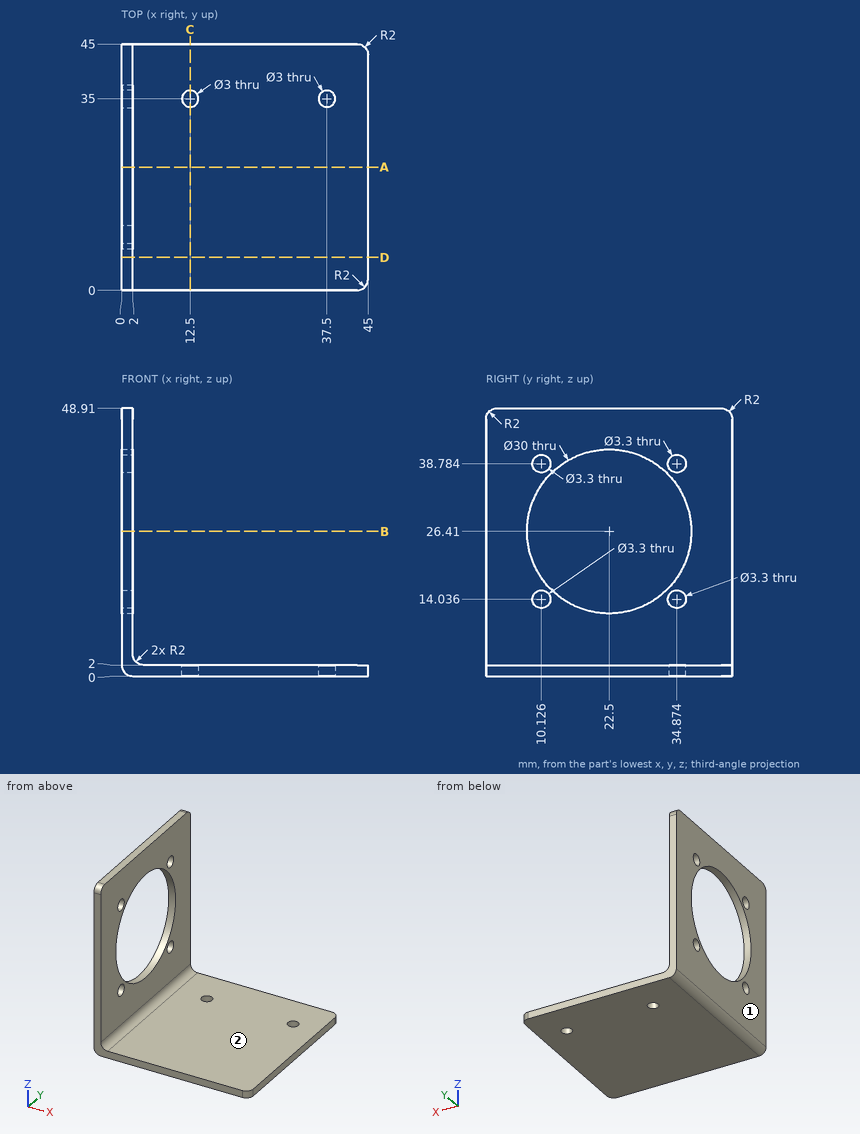
For this review, use the dimensioned drawing (mm, ordinates from the lowest corner) and the shaded views. A direction names the side the tool comes from. Give positions to 0.01 mm unless a question says otherwise; leave off trailing zeros. Loops run counter-clockwise (first coordinate to the right, second up) from the corner with the lowest first, then second, coordinate; pieces in that order, holes last. Notation, with made-up numbers: (22, -30.75) -> (74, -30.75) arc R19 ccw to (74, -14.75) -> close; hole circle Ø2 at (-2.75, -9.75). An arc over 180 degrees is marked (long way). One line per question, with ' | ' between items. Start each with the question number.
(1) We need section B-B (z = 26.41). State the section outline as (x, y) points, and give its area (3 significant figures).
(2) We need section C-C (x = 12.5). State the section outline as (y, z) points.
(3) For the marked faces 1 and 2, list the 3-axis set-ups (+Z, -Z, +X, -X, +Y, -Y) from which the entire face can be reached by the end or side of a thin tool; tool diameter is ignored.
(4) We need section A-A (y = 22.5). State the section outline as (x, z) points, and give its area (3 significant figures).
(5) We need section D-D (y = 6). State the section outline as (x, z) points, and give its area (3 significant figures).
(6) For line 1 (Y direction, x = 37.5, z = 0.7); line 2 (X direction, y = 8, z = 41), list the stretches that pass through material, from the lowest coordinate up.
(7) Insertion check: P1, Ø3, axis at y = 34.87, z = 38.78, coming from the +X side; P2, Ø2, axis at x = 20.5, y = 14, coming from the +Z side; P3, Ø4.5, axis at y = 34.87, z = 14.04, coming from the +X side; P4, Ø12, axis at x = 21, y = 38.5, coming from the -Z side. Each pin has a flat end and moves straight along its axis. Give the tip position at first contact, or say it passes through.
The answers:
1) outline: (0, 0) -> (2, 0) -> (2, 7.5) -> (0, 7.5) -> close; (0, 37.5) -> (2, 37.5) -> (2, 45) -> (0, 45) -> close | area: 30.0 mm^2
2) outline: (0, 0) -> (33.5, 0) -> (33.5, 2) -> (0, 2) -> close; (36.5, 0) -> (45, 0) -> (45, 2) -> (36.5, 2) -> close
3) face 1: +Z, -Z, -X, +Y, -Y | face 2: +Z, +X, +Y, -Y
4) outline: (0, 2) arc R2 ccw to (2, 0) -> (45, 0) -> (45, 2) -> (4, 2) arc R2 cw to (2, 4) -> (2, 11.41) -> (0, 11.41) -> close; (0, 41.41) -> (2, 41.41) -> (2, 48.91) -> (0, 48.91) -> close | area: 124 mm^2
5) outline: (0, 2) arc R2 ccw to (2, 0) -> (45, 0) -> (45, 2) -> (4, 2) arc R2 cw to (2, 4) -> (2, 48.91) -> (0, 48.91) -> close | area: 184 mm^2
6) line 1: y = 0 to 33.5, 36.5 to 45 | line 2: x = 0 to 2
7) P1: passes through | P2: stops at z = 2 | P3: stops at x = 2 | P4: stops at z = 0
